Print and shaded views of the part. All mm, measured from the part's lowest x, y and z. A direction names the side the tool comes from. Round coordinates to 2 decimals unless told otherwise and drop trailing zeros. Loops run counter-clockwise (first coordinate to the right, second up) from the corner with the lowest first, then second, coordinate; pieces in that order, holes last. Notation, with made-up numbers: (-40, 62.5) -> (8, 62.5) arc R23 ccw to (8, 97.5) -> close; hole circle Ø10 at (83, -7). An arc over 180 degrees is marked (long way). Answer as CSV lines item,"result".
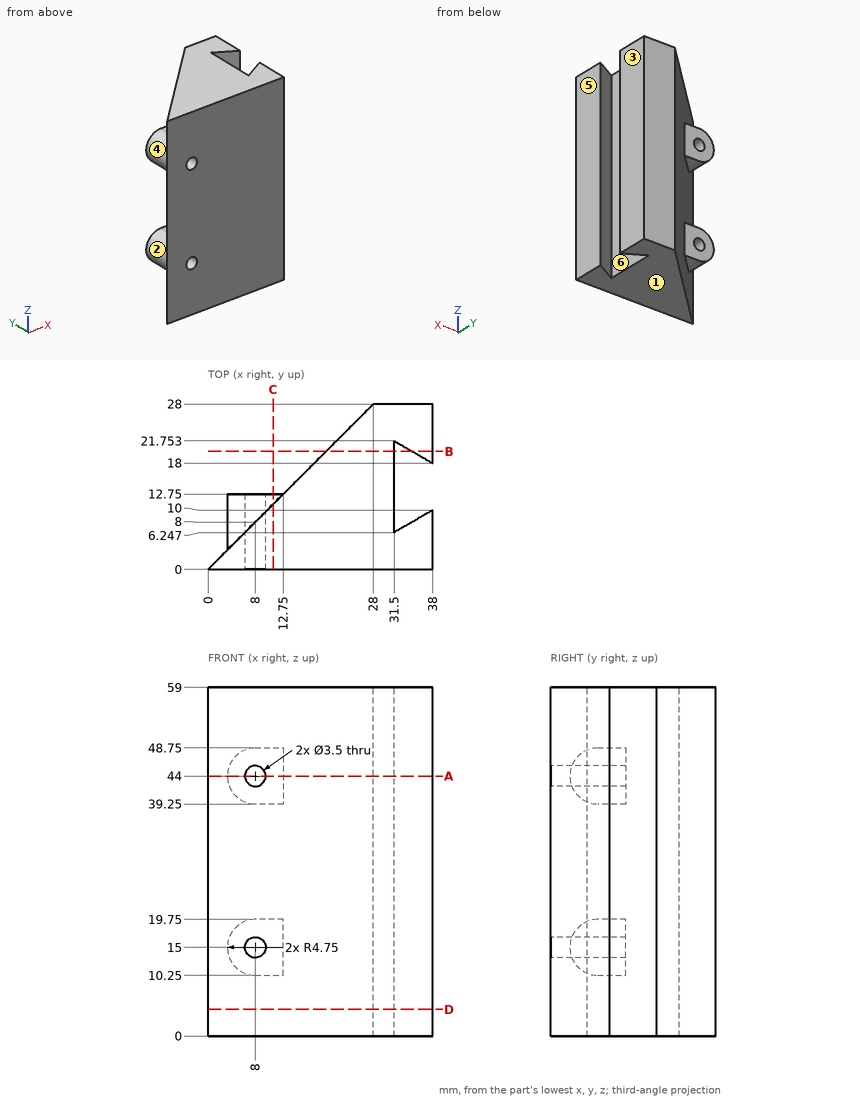
Q1. Drop flat-ended pins along their axis: P1, Ø1.5, axis at y = 17, z = 28.5, coming from the -X side; P2, Ø5.5, axis at x = 8, z = 15, coming from the +Y side; P3, Ø4, axis at x = 10, z = 33.5, coming from the +Y side. Give the stop position or say it passes through.
Geometry results:
P1,"x = 16.25"
P2,"y = 12.75"
P3,"y = 12"
Q2. Saw through at A-A, the plane z = 44. Write the cut outline in (x, y), then the cut area to 3 significant figures.
Geometry results:
outline,"(0, 0) -> (6.25, 0) -> (6.25, 12.75) -> (3.25, 12.75) -> (3.25, 3.25) -> close; (9.75, 0) -> (38, 0) -> (38, 10) -> (31.5, 6.25) -> (31.5, 21.75) -> (38, 18) -> (38, 28) -> (28, 28) -> (12.75, 12.75) -> (9.75, 12.75) -> close"
area,"596 mm2"
Q3. Drill centre lines: line 1 along Z through (x, y) = (8, 9); line 2 along Z through (x, y) = (7.5, 5); line 3 along X through (y, z) = (4.75, 15). Where is each one in solid material? Low to high.
Geometry results:
line 1,"10.25 to 13.25, 16.75 to 19.75, 39.25 to 42.25, 45.75 to 48.75"
line 2,"0 to 13.32, 16.68 to 42.32, 45.68 to 59"
line 3,"3.25 to 6.25, 9.75 to 38"
Q4. Saw through at B-B, the plane y = 20. Write the cut outline in (x, z).
Geometry results:
outline,"(20, 0) -> (31.5, 0) -> (31.5, 59) -> (20, 59) -> close; (34.54, 0) -> (38, 0) -> (38, 59) -> (34.54, 59) -> close"
Q5. Two-plate mould, pull along Z, no slides. Class the marked faces 1, 2 and 3: pulls with the +Z half, pulls with the -Z half, needs draft (parallel to the pull), parting line crosses it, or undercut.
Geometry results:
face 1,"pulls with the -Z half"
face 2,"undercut"
face 3,"needs draft"
Q6. Saw through at C-C, the plane x = 11. Write the cut outline in (y, z).
Geometry results:
outline,"(0, 0) -> (11, 0) -> (11, 10.25) -> (12.75, 10.25) -> (12.75, 19.75) -> (11, 19.75) -> (11, 39.25) -> (12.75, 39.25) -> (12.75, 48.75) -> (11, 48.75) -> (11, 59) -> (0, 59) -> close"
Q7. Saw through at D-D, the plane z = 4.5. Write the cut outline in (x, y), then the cut area to 3 significant figures.
Geometry results:
outline,"(0, 0) -> (38, 0) -> (38, 10) -> (31.5, 6.25) -> (31.5, 21.75) -> (38, 18) -> (38, 28) -> (28, 28) -> close"
area,"596 mm2"
Q8. Which spindle directions (+Z, -Z, +X, -X, +Y, -Y) get a long thin tool onto all of the face, cutting with end or side? Do the marked faces 4, 5 and 6. Say none if no direction does.
Geometry results:
face 4,"-X, +Y"
face 5,"+Z, -Z, +X, +Y, -Y"
face 6,"+Z, -Z"
